from build123d import *

# Parameters (mm, degrees)
SKETCH1_R                = 15.45
SKETCH1_R_2              = 12.45
SKETCH1_R_3              = 33
SKETCH1_R_4              = 30
SKETCH1_R_5              = 4.05
SKETCH1_R_6              = 1.05
BOSS_EXTRUDE2_DEPTH      = 12.4
BOSS_EXTRUDE3_START      = 3
SKETCH2_R                = 33
BOSS_EXTRUDE3_DEPTH      = 3
SKETCH3_R                = 33
SKETCH3_R_2              = 30
BOSS_EXTRUDE4_DEPTH      = 28.6
FILLET1_R                = 10
BOSS_EXTRUDE5_DEPTH      = 12.4
CHAMFER1_SIZE            = 4
FILLET2_R                = 5
BOSS_EXTRUDE6_DEPTH      = 28.6
BOSS_EXTRUDE6_DEPTH_BACK = 14.4
SKETCH5_R                = 4.55
SKETCH5_R_2              = 1.55
FILLET3_R                = 5
CHAMFER2_SIZE            = 2
SKETCH6_W                = 4
SKETCH6_H                = 2
CUT_EXTRUDE1_DEPTH       = 23.4
SKETCH7_R                = 33
SKETCH7_R_2              = 1.55
SKETCH7_R_3              = 6
BOSS_EXTRUDE7_DEPTH      = 3
CUT_EXTRUDE3_START       = -3
SKETCH8_R                = 60.265040847
CUT_EXTRUDE3_DEPTH       = 127
CHAMFER3_SIZE            = 2
CUT_EXTRUDE4_DEPTH       = 10
FILLET4_R                = 2
SKETCH10_R               = 1.1
CUT_EXTRUDE5_DEPTH       = 10
CHAMFER4_SIZE            = 2


with BuildPart() as part:
    # Sketch1 → Boss-Extrude2 (new body)
    # profile 1 of 4: a face of its own
    with BuildSketch(Plane.XY):
        Circle(SKETCH1_R)
        with Locations(Location((0, 0, 0), (0, 0, 180))):
            Circle(SKETCH1_R_2, mode=Mode.SUBTRACT)
    # profile 2 of 4: a face of its own
    with BuildSketch(Plane.XY):
        with Locations(Location((0, 15.45, 0), (0, 0, 180))):
            Circle(SKETCH1_R_3)
        with Locations((0, 15.45)):
            Circle(SKETCH1_R_4, mode=Mode.SUBTRACT)
    # profile 3 of 4: a face of its own
    with BuildSketch(Plane.XY):
        with Locations(Location((11.5, 19.918584287, 0), (0, 0, 180))):
            Circle(SKETCH1_R_5)
        with Locations(Location((11.5, 19.918584287, 0), (0, 0, 180))):
            Circle(SKETCH1_R_6, mode=Mode.SUBTRACT)
    # profile 4 of 4: a face of its own
    with BuildSketch(Plane.XY):
        with Locations(Location((-11.5, 19.918584287, 0), (0, 0, 180))):
            Circle(SKETCH1_R_5)
        with Locations(Location((-11.5, 19.918584287, 0), (0, 0, 180))):
            Circle(SKETCH1_R_6, mode=Mode.SUBTRACT)
    extrude(amount=BOSS_EXTRUDE2_DEPTH)

    # Sketch2 → Boss-Extrude3 (add)
    with BuildSketch(Plane(origin=(0, 0, 0), x_dir=(-1, 0, 0), z_dir=(0, 0, -1)).offset(BOSS_EXTRUDE3_START)):
        with Locations(Location((0, 15.45, 0), (0, 0, 180))):
            Circle(SKETCH2_R)
    extrude(amount=-BOSS_EXTRUDE3_DEPTH)

    # Sketch3 → Boss-Extrude4 (add)
    with BuildSketch(Plane.XY.offset(12.4)):
        with Locations((0, 15.45)):
            Circle(SKETCH3_R)
        with Locations(Location((0, 15.45, 0), (0, 0, 256.137567884))):
            Circle(SKETCH3_R_2, mode=Mode.SUBTRACT)
    extrude(amount=BOSS_EXTRUDE4_DEPTH)

    # Fillet1
    # the kernel refuses this fillet: 10 mm, written as the material it adds along each edge
    with BuildSketch(Plane(origin=(-7.18774525, -13.676213592, 12.4), x_dir=(-0.20848530714015037, 0.9780254990063793, 0), z_dir=(0, 0, -1))) as fillet1_piece_1:
        with BuildLine():
            CenterArc((31.441766058, -6.395526036), FILLET1_R, 140.241533635, 142.62650255)
            ThreePointArc((33.668828933, -16.144381915), (14.016585538, -13.948724396), (0, 0))
            ThreePointArc((0, 0), (11.877146347, -5.568912274), (23.754292694, 0))
        make_face()
    extrude(amount=12.4)
    with BuildSketch(Plane(origin=(7.18774525, -13.676213592, 12.4), x_dir=(0.20848530714015037, 0.9780254990063793, 0), z_dir=(0, 0, -1))) as fillet1_piece_2:
        with BuildLine():
            CenterArc((31.441766058, 6.395526036), FILLET1_R, 77.131963815, 142.62650255)
            ThreePointArc((33.668828933, 16.144381915), (14.016585538, 13.948724396), (0, 0))
            ThreePointArc((0, 0), (11.877146347, 5.568912274), (23.754292694, 0))
        make_face()
    extrude(amount=12.4)

    # Sketch4 → Boss-Extrude5 (add)
    with BuildSketch(Plane.XY):
        Polygon((-15.355968184, 18.680032971), (-12.140166258, 9.556090373), (-4.457434094, 12.838952207), (4.080215127, 12.838952207), (12.140166258, 9.556090373), (15.355968184, 18.680032971), (9.70403689, 17.830268754), (8.160430255, 22.209822799), (0, 15.45), (-8.160430255, 22.209822799), (-10.090971595, 17.830268754), align=None)
    extrude(amount=BOSS_EXTRUDE5_DEPTH)

    # Chamfer1
    chamfer1_edges = [part.edges().sort_by_distance(p)[0] for p in [
        (0, 45.45, 0),
        (-23.339432443, 6.316081984, 0),
        (23.339432443, 6.316081984, 0),
    ]]
    chamfer(chamfer1_edges, length=CHAMFER1_SIZE)

    # Fillet2
    # the kernel refuses this fillet: 5 mm, written as the material it adds along each edge
    with BuildSketch(Plane(origin=(-11.5, 19.918584287, 0), x_dir=(0.4626548968458433, -0.8865384630260337, 0), z_dir=(0.8865384630260337, 0.4626548968458433, 0))) as fillet2_piece_1:
        with BuildLine():
            CenterArc((4.05 + FILLET2_R, -FILLET2_R), FILLET2_R, 90, 90)
            Line((4.05, -FILLET2_R), (4.05, 0))
            Line((4.05, 0), (4.05 + FILLET2_R, 0))
        make_face()
    revolve(axis=Axis((-11.5, 19.918584287, 0), (0, 0, -1)), revolution_arc=359.64)
    with BuildSketch(Plane(origin=(11.5, 19.918584287, 0), x_dir=(-0.4682160132284685, -0.8836140361925214, 0), z_dir=(0.8836140361925214, -0.4682160132284685, 0))) as fillet2_piece_2:
        with BuildLine():
            CenterArc((4.05 + FILLET2_R, -FILLET2_R), FILLET2_R, 90, 90)
            Line((4.05, -FILLET2_R), (4.05, 0))
            Line((4.05, 0), (4.05 + FILLET2_R, 0))
        make_face()
    revolve(axis=Axis((11.5, 19.918584287, 0), (0, 0, -1)), revolution_arc=359.64)

    # Sketch5 → Boss-Extrude6 (add, two sides: drawn at the far end of the back side and taken through both)
    # profile 1 of 3: a face of its own
    with BuildSketch(Plane.XY.offset(12.4).offset(-BOSS_EXTRUDE6_DEPTH_BACK)):
        with Locations((0, 43.45)):
            Circle(SKETCH5_R)
        with Locations((0, 43.45)):
            Circle(SKETCH5_R_2, mode=Mode.SUBTRACT)
    # profile 2 of 3: a face of its own
    with BuildSketch(Plane.XY.offset(12.4).offset(-BOSS_EXTRUDE6_DEPTH_BACK)):
        with Locations((24.248711306, 1.45)):
            Circle(SKETCH5_R)
        with Locations((24.248711306, 1.45)):
            Circle(SKETCH5_R_2, mode=Mode.SUBTRACT)
    # profile 3 of 3: a face of its own
    with BuildSketch(Plane.XY.offset(12.4).offset(-BOSS_EXTRUDE6_DEPTH_BACK)):
        with Locations((-24.248711306, 1.45)):
            Circle(SKETCH5_R)
        with Locations((-24.248711306, 1.45)):
            Circle(SKETCH5_R_2, mode=Mode.SUBTRACT)
    extrude(amount=BOSS_EXTRUDE6_DEPTH + BOSS_EXTRUDE6_DEPTH_BACK)

    # Fillet3
    fillet3_edges = [part.edges().sort_by_distance(p)[0] for p in [
        (23.612570286, -3.055310711, 26.7),
        (27.832354323, 4.25356964, 26.7),
        (-27.832354323, 4.25356964, 26.7),
        (-23.612570286, -3.055310711, 26.7),
        (4.219784038, 45.151741071, 22.5),
        (-4.219784038, 45.151741071, 22.5),
    ]]
    fillet(fillet3_edges, radius=FILLET3_R)

    # Chamfer2
    chamfer2_edges = [part.edges().sort_by_distance(p)[0] for p in [
        (-33, 15.45, -3),
    ]]
    chamfer(chamfer2_edges, length=CHAMFER2_SIZE)

    # Sketch6 → Cut-Extrude1 (cut)
    with BuildSketch(Plane.XY.offset(12.4)):
        with Locations((0, -13.034949107)):
            Rectangle(SKETCH6_W, SKETCH6_H)
    extrude(amount=-CUT_EXTRUDE1_DEPTH, mode=Mode.SUBTRACT)

    # Sketch7 → Boss-Extrude7 (add)
    with BuildSketch(Plane.XY.offset(41)):
        with Locations((0, 15.45)):
            Circle(SKETCH7_R)
        with Locations((-24.248711306, 1.45)):
            Circle(SKETCH7_R_2, mode=Mode.SUBTRACT)
        with Locations((24.248711306, 1.45)):
            Circle(SKETCH7_R_2, mode=Mode.SUBTRACT)
        with Locations((0, 43.45)):
            Circle(SKETCH7_R_2, mode=Mode.SUBTRACT)
        with Locations((11.5, 19.918584287)):
            Circle(SKETCH7_R_3, mode=Mode.SUBTRACT)
    extrude(amount=BOSS_EXTRUDE7_DEPTH)

    # Sketch8 → Cut-Extrude3 (cut)
    with BuildSketch(Plane.XY.offset(44).offset(CUT_EXTRUDE3_START)):
        with Locations((3.003651401, 17.042715902)):
            Circle(SKETCH8_R)
    extrude(amount=-CUT_EXTRUDE3_DEPTH, mode=Mode.SUBTRACT)

    # Chamfer3
    chamfer3_edges = [part.edges().sort_by_distance(p)[0] for p in [
        (-33, 15.45, 44),
    ]]
    chamfer(chamfer3_edges, length=CHAMFER3_SIZE)

    # Sketch9 → Cut-Extrude4 (cut)
    with BuildSketch(Plane.XY.offset(44)):
        with BuildLine():
            ThreePointArc((17.542861073, 29.835702421), (-2.638036688, 37.983112773), (-20.39130231, 25.394606522))
            Line((-20.39130231, 25.394606522), (17.542861073, 29.835702421))
        make_face()
        with BuildLine():
            Line((22.432842806, 12.063560512), (-22.43109496, 12.052002402))
            ThreePointArc((-22.43109496, 12.052002402), (0.00584476, -7.23700894), (22.432842806, 12.063560512))
        make_face()
    extrude(amount=-CUT_EXTRUDE4_DEPTH, mode=Mode.SUBTRACT)

    # Fillet4
    fillet4_edges = [part.edges().sort_by_distance(p)[0] for p in [
        (17.542861073, 29.835702421, 42.5),
        (-20.39130231, 25.394606522, 42.5),
        (-22.43109496, 12.052002402, 42.5),
        (22.432842806, 12.063560512, 42.5),
    ]]
    fillet(fillet4_edges, radius=FILLET4_R)

    # Sketch10 → Cut-Extrude5 (cut)
    with BuildSketch(Plane.XY.offset(44)):
        with Locations((-11.5, 19.918584287)):
            Circle(SKETCH10_R)
    extrude(amount=-CUT_EXTRUDE5_DEPTH, mode=Mode.SUBTRACT)

    # Chamfer4
    # the kernel refuses this chamfer: 2 mm, written as the material it takes off along each edge
    with BuildSketch(Plane(origin=(0, 43.45, 44), x_dir=(1, 0, 0), z_dir=(0, -1, 0))) as chamfer4_piece_1:
        Polygon((1.55, -CHAMFER4_SIZE), (1.55 + CHAMFER4_SIZE, 0), (1.55, 0), align=None)
    revolve(axis=Axis((0, 43.45, 44), (0, 0, 1)), mode=Mode.SUBTRACT)
    with BuildSketch(Plane(origin=(-24.248711306, 1.45, 44), x_dir=(1, 0, 0), z_dir=(0, -1, 0))) as chamfer4_piece_2:
        Polygon((1.55, -CHAMFER4_SIZE), (1.55 + CHAMFER4_SIZE, 0), (1.55, 0), align=None)
    revolve(axis=Axis((-24.248711306, 1.45, 44), (0, 0, 1)), mode=Mode.SUBTRACT)
    with BuildSketch(Plane(origin=(24.248711306, 1.45, 44), x_dir=(1, 0, 0), z_dir=(0, -1, 0))) as chamfer4_piece_3:
        Polygon((1.55, -CHAMFER4_SIZE), (1.55 + CHAMFER4_SIZE, 0), (1.55, 0), align=None)
    revolve(axis=Axis((24.248711306, 1.45, 44), (0, 0, 1)), mode=Mode.SUBTRACT)


solid = part.part
The listing builds one solid part. Answer for the finished solid, in the listing's coordinates (mm). A direction names the side the tool comes from. Round coordinates to 2 decimals unless told otherwise and drop trailing zeros. Order: outer loops, then holes, each group sorted by start corner. A loop starts at its lowest first (then second) coordinate and runs counter-clockwise, first axis right, second up. Notation, with made-up numbers: M 86.25,21.5 L 143.25,21.5 A17 cw 143.25,34.5 Z; hole C -14.5,15.5 d6. An arc over 180 degrees is marked long. Answer in a Markdown table with one row per item. Add a question column.
1) The part is cut by section A-A on z = 42.45. Determine the outline of the cut face in (x, y).
2) Determine the mould class of faces 1 (the face through (-1.63, 27.59, 42.52)), 2 (the face through (-7.154, -16.765, 41.493)), 3 (the face through (0, 16, 41)) for opening direction Y: pulls with the +Y half, pulls with the -Y half, needs draft (parallel to the pull), parting line crosses it, or undercut.
3) The part is cut by section D-D on x = 10.5. Count the separate pieces of the cut face and the enclosed holes in it, plus the area to 3 significant figures.
4) Flat-ended cylindrical pins translate along their axes: pin 1 Ø5 at (x, y) = (0, 43.45) entering from +Z; pin 2 Ø3.5 at (x, y) = (-11.5, 19.92) entering from -Z; pin 3 Ø2.5 at (x, y) = (24.25, 1.45) entering from +Z; pin 4 Ø4 at (x, y) = (-24.25, 1.45) entering from +Z. Find the tip coordinate at first contact, or state that the pin passes through.
5) The part is cut by section B-B on y = 15.45. Determine the outline of the cut face in (x, z).
6) Consider line 1 along Y through (x, z) = (0, 41.55); line 2 along X through (y, z) = (2, 41.65); line 3 along Y through (x, z) = (-5.5, 41.8). Determine where each line is inside the solid, lowest interval first. Write a range as from..to.
7) Which of the six approach directions +Z, -Z, +X, -X, +Y, -Y give full straight-line access (tool end or side, diameter ignored) to faces 4 (the face through (23.014, 2.582, 42.125)), 5 (the face through (-0.409, -7.233, 42.521))?
8) The part is cut by section C-C on x = 0. Determine the outline of the cut face in (y, z) (3 decimals).
Findings below:
| question | item | result |
|---|---|---|
| 1 | outline | C 0,15.45 d65.1; hole C -24.25,1.45 d4; hole M -21.9,9.53 A22.69 ccw 21.9,9.54 A2 ccw 19.97,12.06 L -19.97,12.05 A2 ccw Z; hole M -18.15,29.06 A2 ccw -16.32,25.87 L 13.47,29.36 A2 ccw 14.52,32.88 A22.69 ccw Z; hole C -11.5,19.92 d2.2; hole C 0,43.45 d4; hole C 11.5,19.92 d12; hole C 24.25,1.45 d4 |
| 2 | face 1 | undercut |
| 2 | face 2 | parting line crosses it |
| 2 | face 3 | needs draft |
| 3 | separate pieces | 4 |
| 3 | enclosed holes | 0 |
| 3 | area | 78.2 mm² |
| 4 | pin 1 | stops at z = 42.95 |
| 4 | pin 2 | stops at z = 41 |
| 4 | pin 3 | passes through |
| 4 | pin 4 | stops at z = 42.45 |
| 5 | outline | M -33,41 L 7.5,41 L 7.5,44 L -31,44 L -33,42 Z; M 15.5,41 L 33,41 L 33,42 L 31,44 L 15.5,44 Z |
| 6 | line 1 | y = -17.55..-7.24, 12.06..27.78, 38.14..41.9, 45..48.45 |
| 6 | line 2 | x = -30.13..-25.7, -22.8..-18.27, 18.27..22.8, 25.7..30.13 |
| 6 | line 3 | y = -17.09..-6.56, 12.06..27.14, 37.46..47.99 |
| 7 | face 4 | +Z |
| 7 | face 5 | +Z, -Z |
| 8 | outline | M -17.55,41 L -7.237,41 L -7.237,44 L -15.55,44 L -17.55,42 Z; M 12.058,41 L 27.782,41 L 27.782,44 L 12.058,44 Z; M 38.137,41 L 41.9,41 L 41.9,42 L 39.9,44 L 38.137,44 Z; M 45,41 L 48.45,41 L 48.45,42 L 46.725,43.725 L 45,42 Z |
